Verification items for the finished model (mm, model axes). Face numbers are marked on the shaded views. A direction names the side the tool comes from. Give positions to 0.01 mm unless a question says otherwise; leave off trailing zeros. Order: outer loops, then holes, each group sorted by start corner. A loop starts at its lowest first (then second) coordinate and runs counter-clockwise, first axis right, second up. Notation, with made-up numbers: (57, 36.25) -> (83, 36.25) arc R20 ccw to (83, 58.25) -> close; hole circle Ø5 at (-11.75, 14). An arc over 180 degrees is marked (long way). Return JSON: item names as keys, results as strings. Group by question number.
(1) Cross-section at D-D on x = 6. Enter the section's corners in (y, z).
(2) Cross-section at A-A on z = 0. Enter the section's corners in (x, y) (3 decimals).
(3) Cross-section at B-B on y = 4.2. Enter the section's corners in (x, z) (3 decimals), then the cut area to 3 significant figures.
(4) Tool access check on the marked faces 1 and 2. Record the directions out of +Z, -Z, +X, -X, +Y, -Y that give a thin tool (end or side, any length) a straight path to the whole face; none if there is none.
(5) Release check for a two-part mould opening along Z. For the marked faces 3, 4, 5 and 6 record: pulls with the +Z half, pulls with the -Z half, needs draft (parallel to the pull), parting line crosses it, or undercut.
(6) Cross-section at C-C on x = 0. Enter the section's corners in (y, z) (3 decimals).
(7) Depth check by flat-ended pin: pin 1 Ø6.5 at (x, z) = (0, 0) entering from +Y; pin 2 Ø1 at (x, y) = (4.5, 3) entering from +Z; pin 3 Ø2.5 at (x, z) = (-3.5, -1.5) entering from +Y. Enter the tip coordinate at first touch or a pass-through.
(8) Thickness scan on line 1 along Z through (x, y) = (-2.75, 0.2); line 2 along Y through (x, z) = (2.25, 3); line 3 along Z through (x, y) = (-6.5, 2.7). Record the ranges inside material, lowest first.
from build123d import *

# Parameters (mm, degrees)
SKETCH1_R                       = 10
BOSS_EXTRUDE1_DEPTH             = 5
TAP_DRILL_FOR_M3X0_5_TAP1_D     = 2.5
TAP_DRILL_FOR_M3X0_5_TAP1_DEPTH = 38.1
CIRPATTERN1_COUNT               = 4
F_14_0_182_DIAMETER_HOLE1_D     = 7.1499984
CUT_EXTRUDE2_DEPTH              = 3.1


with BuildPart() as part:
    # Sketch1 → Boss-Extrude1 (new body)
    with BuildSketch(Plane(origin=(0, 0, 0), x_dir=(1, 0, 0), z_dir=(0, 1, 0))):
        Circle(SKETCH1_R)
    extrude(amount=BOSS_EXTRUDE1_DEPTH)

    # Tap Drill for M3x0.5 Tap1
    with Locations(Plane(origin=(0, 5, 0), x_dir=(1, 0, 0), z_dir=(0, 1, 0))):
        with Locations((7, 0)):
            tap_drill_for_m3x0_5_tap1 = Hole(TAP_DRILL_FOR_M3X0_5_TAP1_D / 2, depth=TAP_DRILL_FOR_M3X0_5_TAP1_DEPTH)

    # CirPattern1: Tap Drill for M3x0.5 Tap1 ×4 about axis, 1 skipped
    cirpattern1_axis = Axis((0, 0, 0), (0, -1, 0))
    add([tap_drill_for_m3x0_5_tap1.rotate(cirpattern1_axis, i * 360 / CIRPATTERN1_COUNT) for i in range(1, CIRPATTERN1_COUNT) if i not in (2,)], mode=Mode.SUBTRACT)

    # 14 _0.182_ Diameter Hole1 (through all)
    with Locations(Plane(origin=(0, 5, 0), x_dir=(1, 0, 0), z_dir=(0, 1, 0))):
        with Locations((0, 0)):
            Hole(F_14_0_182_DIAMETER_HOLE1_D / 2)

    # Sketch9 → Cut-Extrude2 (cut)
    with BuildSketch(Plane(origin=(0, 5, 0), x_dir=(1, 0, 0), z_dir=(0, 1, 0))):
        with BuildLine():
            Line((-0.518585505, 3.739209547), (-12.660050371, 2.055327537))
            ThreePointArc((-12.660050371, 2.055327537), (-14.45, 0), (-12.660050371, -2.055327537))
            Line((-12.660050371, -2.055327537), (-0.518585505, -3.739209547))
            ThreePointArc((-0.518585505, -3.739209547), (3.7749992, 0), (-0.518585505, 3.739209547))
        make_face()
    extrude(amount=-CUT_EXTRUDE2_DEPTH, mode=Mode.SUBTRACT)


solid = part.part
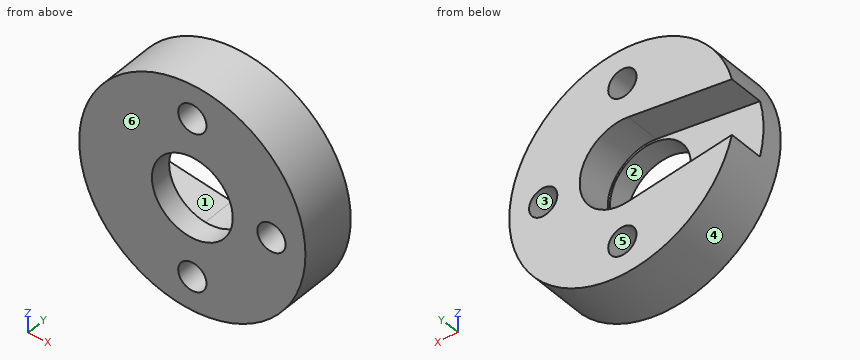
Verdict:
{
 "1": {"outline": "(0, -8) -> (5, -8) -> (5, -0.75) -> (0, -0.75) -> close; (0, 0.75) -> (5, 0.75) -> (5, 8) -> (0, 8) -> close"},
 "2": {"outline": "(-10, 0) -> (-3.575, 0) -> (-3.575, 1.9) -> (-10, 1.9) -> close; (3.575, 0) -> (5.75, 0) -> (5.75, 5) -> (3.775, 5) -> (3.775, 1.9) -> (3.575, 1.9) -> close; (8.25, 0) -> (10, 0) -> (10, 5) -> (8.25, 5) -> close"},
 "3": {"outline": "(-9.691, -2.467) arc R10 ccw (long way) to (-9.691, 2.467) -> (-0.519, 3.739) arc R3.775 cw (long way) to (-0.519, -3.739) -> close; hole circle Ø2.5 at (0, -7); hole circle Ø2.5 at (0, 7); hole circle Ø2.5 at (7, 0)", "area": "215 mm²"},
 "4": {"face 1": "+Y", "face 2": "+Y, -Y"},
 "5": {"face 3": "undercut", "face 4": "parting line crosses it", "face 5": "undercut", "face 6": "needs draft"},
 "6": {"outline": "(0, -10) -> (5, -10) -> (5, -8.25) -> (0, -8.25) -> close; (0, -5.75) -> (5, -5.75) -> (5, -3.775) -> (1.9, -3.775) -> (1.9, -3.575) -> (0, -3.575) -> close; (0, 3.575) -> (1.9, 3.575) -> (1.9, 3.775) -> (5, 3.775) -> (5, 5.75) -> (0, 5.75) -> close; (0, 8.25) -> (5, 8.25) -> (5, 10) -> (0, 10) -> close"},
 "7": {"pin 1": "through", "pin 2": "z = 9.17", "pin 3": "y = 1.9"},
 "8": {"line 1": "-9.61 to -2.28, 2.28 to 9.61", "line 2": "0 to 1.9", "line 3": "-7.6 to -2.91, 2.91 to 7.6"}
}
